```python
from build123d import *

# Parameters (mm, degrees)
F0_W     = 91.358508
F0_H     = 107.0102
F0_W_2   = 68.661492
F1_DEPTH = 25.4
F2_T     = -2.54
F3_W     = 68.661492
F3_H     = 25.4
F4_DEPTH = 31.496


with BuildPart() as f1:
    # F0 (on Front) → F1 (new body)
    with BuildSketch(Plane.XZ):
        with Locations((-45.679254, -5.917441)):
            Rectangle(F0_W, F0_H)
        with Locations((34.330746, -5.917441)):
            Rectangle(F0_W_2, F0_H)
    extrude(amount=F1_DEPTH)

    # F2
    f2_openings = [f1.faces().sort_by_distance(p)[0] for p in [
        (-11.348508, -25.4, -5.917441),
    ]]
    offset(amount=F2_T, openings=f2_openings)

    # F3 (on face) → F4 (cut, symmetric)
    with BuildSketch(Plane(origin=(0, 0, -59.422541), x_dir=(1, 0, 0), z_dir=(0, 0, -1))):
        with Locations((34.330746, 12.7)):
            Rectangle(F3_W, F3_H)
    extrude(amount=F4_DEPTH, both=True, mode=Mode.SUBTRACT)


solid = f1.part
```
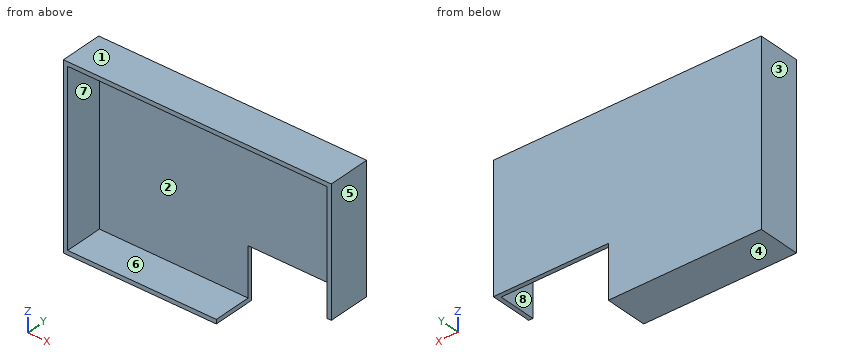
The model under review builds one solid part; all positions refer to its coordinate system, in mm. Face numbers are marked on the shaded views. A direction names the side the tool comes from. Give positions to 0.01 mm unless a question says otherwise; leave off trailing zeros. Loops run counter-clockwise (first coordinate to the right, second up) from the corner with the lowest first, then second, coordinate; pieces in that order, holes last. Notation, with made-up numbers: (81.25, -0.75) - (114.25, -0.75) arc R13 cw to (114.25, 4.25) - close; hole circle Ø4 at (-29, -2). An arc over 180 degrees is marked (long way). Answer as a JSON object with one key per item and string values.
Q1. For the marked faces 5, 6, 7 and 8, list the 3-axis set-ups (+Z, -Z, +X, -X, +Y, -Y) from which the entire face can be reached by the end or side of a thin tool; tool diameter is ignored.
Worked out:
{"face 5": "+Z, -Z, +X, +Y, -Y", "face 6": "+X, -Y", "face 7": "-Y", "face 8": "-Z, -Y"}
Q2. Add section C-C on x = -10.5. State the section outline as (y, z) points, plus the area to 3 significant figures.
Worked out:
{"outline": "(-25.4, -59.42) - (0, -59.42) - (0, 47.59) - (-25.4, 47.59) - (-25.4, 45.05) - (-2.54, 45.05) - (-2.54, -56.88) - (-25.4, -56.88) - close", "area": "388 mm^2"}
Q3. Mouldability with a two-part tool opening along Z and no side actions: class the marked faces 1, 2, 3 and 4 as +Z half, -Z half, draft (parallel to the pull), parting line (faces both ways), or undercut.
Worked out:
{"face 1": "+Z half", "face 2": "undercut", "face 3": "draft", "face 4": "-Z half"}
Q4. Add section A-A on z = 32. State the section outline as (x, y) points.
Worked out:
{"outline": "(-91.36, -25.4) - (-88.82, -25.4) - (-88.82, -2.54) - (66.12, -2.54) - (66.12, -25.4) - (68.66, -25.4) - (68.66, 0) - (-91.36, 0) - close"}
Q5. Insertion check: pin 1 (5 mm diameter, centred on y = -19.5, z = -38, fed in from +X); pin 2 (2 mm diameter, centred on x = -6.5, z = -47.5, fed in from -Y); pin 3 (10 mm diameter, centred on x = 40, y = -20, fed in from -Z). Each pin has a flat end and moves straight along its axis. Give the tip position at first contact, or say it passes through.
Worked out:
{"pin 1": "stops at x = -88.82", "pin 2": "stops at y = -2.54", "pin 3": "stops at z = 45.05"}
Q6. Add section D-D on z = -30.5. State the section outline as (x, y) points.
Worked out:
{"outline": "(-91.36, -25.4) - (-88.82, -25.4) - (-88.82, -2.54) - (0, -2.54) - (0, 0) - (-91.36, 0) - close"}
Q7. Add section B-B on y = -12.25. State the section outline as (x, z) points, plus the area to 3 significant figures.
Worked out:
{"outline": "(-91.36, -59.42) - (0, -59.42) - (0, -56.88) - (-88.82, -56.88) - (-88.82, 45.05) - (66.12, 45.05) - (66.12, -27.93) - (68.66, -27.93) - (68.66, 47.59) - (-91.36, 47.59) - close", "area": "1,080 mm^2"}
Q8. To check wall thickness, follow line 1 along Z through (x, y) = (-19, -14.5); line 2 along X through (y, z) = (-17.75, 14.5); line 3 along Y through (x, z) = (-23.5, -39). State the ranges of each line that lie inside material, in increasing order.
Worked out:
{"line 1": "z = -59.42 to -56.88, 45.05 to 47.59", "line 2": "x = -91.36 to -88.82, 66.12 to 68.66", "line 3": "y = -2.54 to 0"}
